The model under review builds one solid part; all positions refer to its coordinate system, in mm. Face numbers are marked on the shaded views. A direction names the side the tool comes from. Coordinates: 2 decimals unless noted, no trailing zeros. Loops run counter-clockwise (first coordinate to the right, second up) from the corner with the lowest first, then second, coordinate; pieces in that order, holes last. Notation, with made-up numbers: M -30.75,19 L 8.25,19 A21 ccw 8.25,36 Z; hole C 56.25,85.25 d9. An arc over 180 degrees is marked long. One line per item, written item: value.
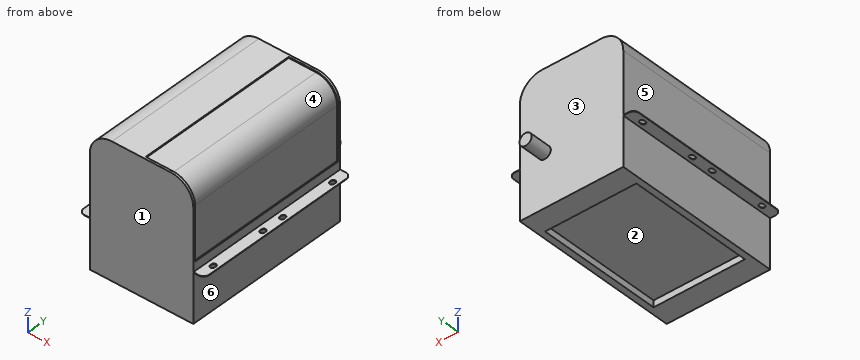
```python
from build123d import *

# Parameters (mm, degrees)
F1_DEPTH  = 76.5
F2_W      = 113.5
F2_H      = 0.5
F3_DEPTH  = 153
F4_R      = 5
F6_DEPTH  = 44.501
F7_R      = 5.5
F8_DEPTH  = 20
F9_W      = 82.5
F9_H      = 113
F10_DEPTH = 6
F12_START = -2
F12_DEPTH = 149


with BuildPart() as f1:
    # F0 (on Front) → F1 (new body, symmetric)
    with BuildSketch(Plane.XZ):
        with BuildLine():
            ThreePointArc((46.75, 40), (12.6078643763, 25.8578643763), (26.75, 60))
            Line((26.75, 60), (-26.75, 60))
            ThreePointArc((-26.75, 60), (-12.6078643763, 54.1421356237), (-6.75, 40))
            ThreePointArc((-6.75, 40), (-26.75, 20), (-46.75, 40))
            Line((-46.75, 40), (-46.75, -60))
            Line((-46.75, -60), (46.75, -60))
            Line((46.75, -60), (46.75, 40))
        make_face()
        with BuildLine():
            ThreePointArc((46.75, 40), (40.8921356237, 54.1421356237), (26.75, 60))
            ThreePointArc((26.75, 60), (12.6078643763, 25.8578643763), (46.75, 40))
        make_face()
        with BuildLine():
            ThreePointArc((-6.75, 40), (-12.6078643763, 54.1421356237), (-26.75, 60))
            ThreePointArc((-26.75, 60), (-40.8921356237, 54.1421356237), (-46.75, 40))
            ThreePointArc((-46.75, 40), (-26.75, 20), (-6.75, 40))
        make_face()
    extrude(amount=F1_DEPTH, both=True)

    # F2 (on face) → F3 (join, through all)
    with BuildSketch(Plane.XZ.offset(76.5)):
        with Locations((0, -15.75)):
            Rectangle(F2_W, F2_H)
    extrude(amount=-F3_DEPTH)

    # F4
    f4_edges = [f1.edges().sort_by_distance(p)[0] for p in [
        (56.75, 76.5, -15.75),
        (-56.75, 76.5, -15.75),
        (-56.75, -76.5, -15.75),
        (56.75, -76.5, -15.75),
    ]]
    fillet(f4_edges, radius=F4_R)

    # F5 (on face) → F6 (cut, through all)
    with BuildSketch(Plane.XY.offset(-15.5)):
        with BuildLine():
            ThreePointArc((-49.7, 62.95), (-51.75, 65), (-53.8, 62.95))
            Line((-53.8, 62.95), (-53.8, 61.45))
            ThreePointArc((-53.8, 61.45), (-51.75, 59.4), (-49.7, 61.45))
            Line((-49.7, 61.45), (-49.7, 62.95))
        make_face()
        with BuildLine():
            ThreePointArc((-49.7, 11.05), (-51.75, 13.1), (-53.8, 11.05))
            Line((-53.8, 11.05), (-53.8, 9.55))
            ThreePointArc((-53.8, 9.55), (-51.75, 7.5), (-49.7, 9.55))
            Line((-49.7, 9.55), (-49.7, 11.05))
        make_face()
        with BuildLine():
            ThreePointArc((54.3, 62.95), (52.25, 65), (50.2, 62.95))
            Line((50.2, 62.95), (50.2, 61.45))
            ThreePointArc((50.2, 61.45), (52.25, 59.4), (54.3, 61.45))
            Line((54.3, 61.45), (54.3, 62.95))
        make_face()
        with BuildLine():
            ThreePointArc((54.3, 11.05), (52.25, 13.1), (50.2, 11.05))
            Line((50.2, 11.05), (50.2, 9.55))
            ThreePointArc((50.2, 9.55), (52.25, 7.5), (54.3, 9.55))
            Line((54.3, 9.55), (54.3, 11.05))
        make_face()
        with BuildLine():
            Line((-49.7, -62.95), (-49.7, -61.45))
            ThreePointArc((-49.7, -61.45), (-51.75, -59.4), (-53.8, -61.45))
            Line((-53.8, -61.45), (-53.8, -62.95))
            ThreePointArc((-53.8, -62.95), (-51.75, -65), (-49.7, -62.95))
        make_face()
        with BuildLine():
            Line((-53.8, -9.55), (-53.8, -11.05))
            ThreePointArc((-53.8, -11.05), (-51.75, -13.1), (-49.7, -11.05))
            Line((-49.7, -11.05), (-49.7, -9.55))
            ThreePointArc((-49.7, -9.55), (-51.75, -7.5), (-53.8, -9.55))
        make_face()
        with BuildLine():
            Line((54.3, -11.05), (54.3, -9.55))
            ThreePointArc((54.3, -9.55), (52.25, -7.5), (50.2, -9.55))
            Line((50.2, -9.55), (50.2, -11.05))
            ThreePointArc((50.2, -11.05), (52.25, -13.1), (54.3, -11.05))
        make_face()
        with BuildLine():
            Line((54.3, -62.95), (54.3, -61.45))
            ThreePointArc((54.3, -61.45), (52.25, -59.4), (50.2, -61.45))
            Line((50.2, -61.45), (50.2, -62.95))
            ThreePointArc((50.2, -62.95), (52.25, -65), (54.3, -62.95))
        make_face()
    extrude(amount=-F6_DEPTH, mode=Mode.SUBTRACT)

    # F7 (on face) → F8 (join)
    with BuildSketch(Plane(origin=(0, 76.5, 0), x_dir=(-1, 0, 0), z_dir=(0, 1, 0))):
        with Locations((-24.25, -12.5)):
            Circle(F7_R)
    extrude(amount=F8_DEPTH)

    # F9 (on face) → F10 (cut)
    with BuildSketch(Plane(origin=(0, 0, -60), x_dir=(1, 0, 0), z_dir=(0, 0, -1))):
        Rectangle(F9_W, F9_H)
    extrude(amount=-F10_DEPTH, mode=Mode.SUBTRACT)

    # F11 (on face) → F12 (cut)
    with BuildSketch(Plane(origin=(0, 76.5, 0), x_dir=(-1, 0, 0), z_dir=(0, 1, 0)).offset(F12_START)):
        with BuildLine():
            ThreePointArc((-45.75, 40), (-40.1850288425, 53.4350288425), (-26.75, 59))
            Line((-26.75, 59), (-2, 59))
            Line((-2, 59), (-2, 60))
            Line((-2, 60), (-26.75, 60))
            ThreePointArc((-26.75, 60), (-40.8921356237, 54.1421356237), (-46.75, 40))
            Line((-46.75, 40), (-46.75, -7.5))
            Line((-46.75, -7.5), (-45.75, -7.5))
            Line((-45.75, -7.5), (-45.75, 40))
        make_face()
    extrude(amount=-F12_DEPTH, mode=Mode.SUBTRACT)


solid = f1.part
```
(1) Insertion check: pin 1 Ø3 at (x, y) = (-52.5, -4.5) entering from -Z; pin 2 Ø4 at (x, z) = (-10.5, -22) entering from +Y; pin 3 Ø2 at (x, y) = (-3, -1.5) entering from -Z. Each pin has a flat end and moves straight along its axis. Give the tip position at first contact, or say it passes through.
Checks:
pin 1: z = -16
pin 2: y = 76.5
pin 3: z = -54
(2) Add section A-A on x = -9. State the section outline as (y, z) points.
Checks:
outline: M -76.5,-60 L -56.5,-60 L -56.5,-54 L 56.5,-54 L 56.5,-60 L 76.5,-60 L 76.5,60 L -76.5,60 Z
(3) Draft analysis for pull direction Y (two halves, no side actions). For the marked faces 1, 2 and 3, state which applies: pulls with the +Y half, pulls with the -Y half, needs draft (parallel to the pull), parting line crosses it, or undercut.
Checks:
face 1: pulls with the -Y half
face 2: undercut
face 3: pulls with the +Y half
(4) Add section B-B on y = 19. State the section outline as (x, z) points, then the cut area to 3 significant figures.
Checks:
outline: M -56.75,-16 L -46.75,-16 L -46.75,-60 L -41.25,-60 L -41.25,-54 L 41.25,-54 L 41.25,-60 L 46.75,-60 L 46.75,-16 L 56.75,-16 L 56.75,-15.5 L 46.75,-15.5 L 46.75,-7.5 L 45.75,-7.5 L 45.75,40 A19 ccw 26.75,59 L 2,59 L 2,60 L -26.75,60 A20 ccw -46.75,40 L -46.75,-15.5 L -56.75,-15.5 Z
area: 10,500 mm^2
(5) Tool access review of the marked faces 4, 5 and 6: name each direction out of +Z, -Z, +X, -X, +Y, -Y from which nothing blocks a thin tool from reaching the whole face with its end or side.
Checks:
face 4: +Z, +X
face 5: +Z, -X, +Y, -Y
face 6: -Z, +X, +Y, -Y
(6) Add section D-D on x = 32.5. State the section outline as (y, z) points.
Checks:
outline: M -76.5,-60 L -56.5,-60 L -56.5,-54 L 56.5,-54 L 56.5,-60 L 76.5,-60 L 76.5,59.16 L 74.5,59.16 L 74.5,58.11 L -74.5,58.11 L -74.5,59.16 L -76.5,59.16 Z
(7) Add section C-C on z = -12.5. State the section outline as (x, y) points.
Checks:
outline: M -46.75,-76.5 L 46.75,-76.5 L 46.75,76.5 L 29.75,76.5 L 29.75,96.5 L 18.75,96.5 L 18.75,76.5 L -46.75,76.5 Z
(8) To check wall thickness, follow L1, parallel to Z at x = 4, y = 7; L2, parallel to Y at x = -29.5, z = 5.5; L3, parallel to X at y = -19, z = -15. State the ranges of each line that lie inside material, in increasing order. Write a range as [from, to].
Checks:
L1: [-54, 59]
L2: [-76.5, 76.5]
L3: [-46.75, 46.75]
